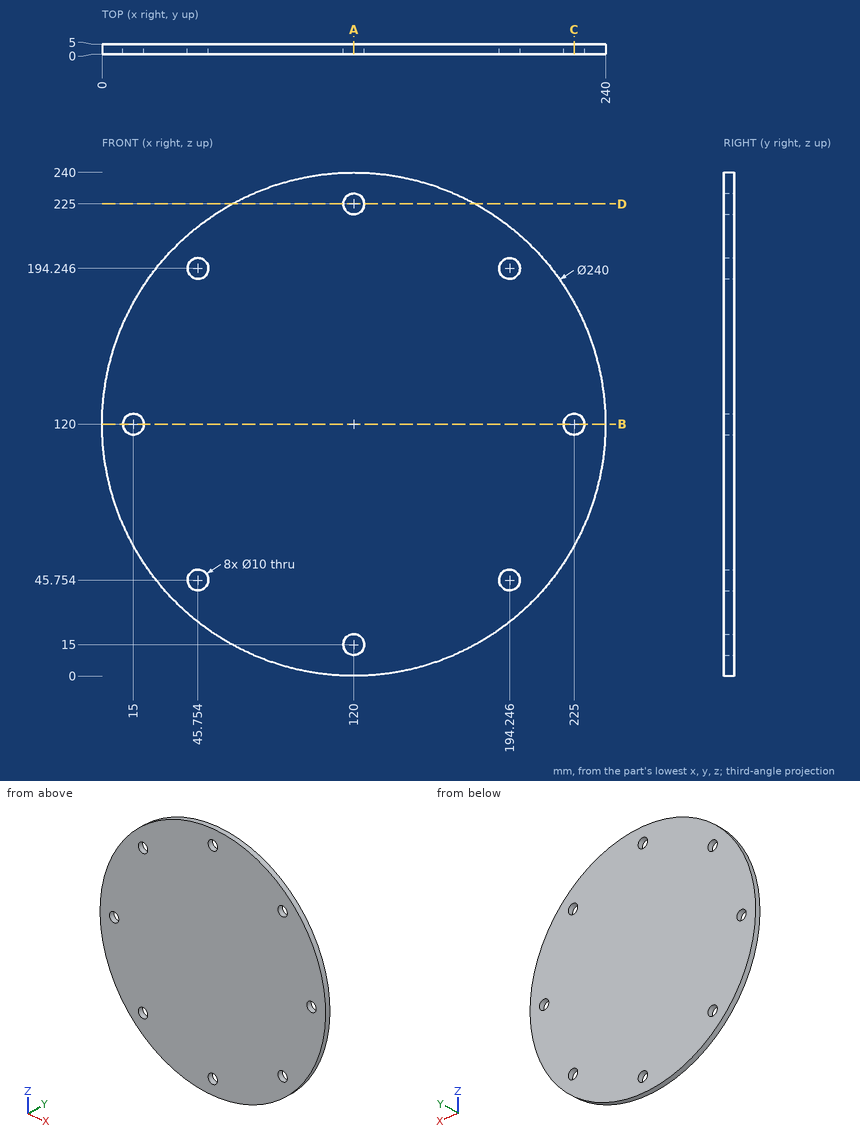
Geometry check sheet. Reference: drawing and pictorial views, mm from the part's lowest x, y, z. Give positions to 0.01 mm unless a question says otherwise; leave off trailing zeros. Order: outer loops, then holes, each group sorted by start corner. A loop starts at its lowest first (then second) coordinate and runs counter-clockwise, first axis right, second up. Notation, with made-up numbers: (60.25, -39) -> (65.25, -39) arc R18 cw to (65.25, -7) -> close; hole circle Ø8 at (-11, -28.75). An arc over 180 degrees is marked (long way). Use CSV: the item, a comma, the result in double quotes. Start each with the question number.
1) Material ranges on line 1 (X direction, y = 2.9, z = 120); line 2 (Z direction, x = 192.5, y = 2.5); line 3 (Z direction, x = 43.5, y = 1.15) (1 decimal), recorded low to high. Write a range as from..to.
2) Go/stop test with flat-tipped pins: P1, Ø3, axis at y = 4.5, z = 212.5, coming from the +X side (1 decimal); P2, Ø1.5, axis at y = 4, z = 68, coming from the -X side (1 decimal); P3, Ø8, axis at x = 45.75, z = 45.75, coming from the -Y side; P4, Ø2, axis at x = 211, y = 3.5, coming from the -Z side. Record where each tip stops, or that it passes through.
3) Sectioned sample at D-D, the plane z = 225. Record the boundary of the cut face in (x, y) (1 decimal).
4) Sectioned sample at A-A, the plane x = 120. Record the boundary of the cut face in (y, z).
5) Sectioned sample at C-C, the plane x = 225. Record the boundary of the cut face in (y, z) (1 decimal), plus the area to 3 significant figures.
6) Sectioned sample at B-B, the plane z = 120. Record the boundary of the cut face in (x, y).
Recorded:
1,line 1,"0..10, 20..220, 230..240"
1,line 2,"24.38..41.07, 50.44..189.56, 198.93..215.62"
1,line 3,"27.5..41.3, 50.2..189.8, 198.7..212.5"
2,P1,"x = 198.2"
2,P2,"x = 11.5"
2,P3,"through"
2,P4,"z = 40.63"
3,outline,"(61.9, 0) -> (115, 0) -> (115, 5) -> (61.9, 5) -> close; (125, 0) -> (178.1, 0) -> (178.1, 5) -> (125, 5) -> close"
4,outline,"(0, 0) -> (5, 0) -> (5, 10) -> (0, 10) -> close; (0, 20) -> (5, 20) -> (5, 220) -> (0, 220) -> close; (0, 230) -> (5, 230) -> (5, 240) -> (0, 240) -> close"
5,outline,"(0, 61.9) -> (5, 61.9) -> (5, 115) -> (0, 115) -> close; (0, 125) -> (5, 125) -> (5, 178.1) -> (0, 178.1) -> close"
5,area,"531 mm2"
6,outline,"(0, 0) -> (10, 0) -> (10, 5) -> (0, 5) -> close; (20, 0) -> (220, 0) -> (220, 5) -> (20, 5) -> close; (230, 0) -> (240, 0) -> (240, 5) -> (230, 5) -> close"
